Work out the finished part from the listing and answer in its coordinate system (mm). Face numbers are marked on the shaded views. A direction names the side the tool comes from. Round coordinates to 2 decimals unless told otherwise and drop trailing zeros. Write each loop counter-clockwise with the first axis right and the second up, starting at its lowest first coordinate (ties: lowest second). Pieces come first, ordered by that corner, then holes. Notation, with made-up numbers: M 49,-1.5 L 80,-1.5 A18 cw 80,9.5 Z; hole C -12,11.5 d10. An arc over 180 degrees is marked long. One line per item, written item: value. Start each with the question number.
Q1. A tool of negligible diameter and unlimited length cuts with its end or side. For the marked faces 1 and 2, from which of +Z, -Z, +X, -X, +Y, -Y can it reach the whole face along a straight path? Write none if from no direction.
Q2. Find section A-A (y = 0). Write down the section's boundary in (x, z) (3 decimals), and give its area (3 significant figures).
Q3. Consider probe 1 along Y at (x, z) = (16.51, 1.2); probe 2 along Z at (x, y) = (13, -4.75); probe 3 along X at (y, z) = (-1.25, 1.25). Determine where each line is inside the solid, lowest interval first.
Q4. Given pin 1 Ø7.5 at (y, z) = (0, 9.525) entering from +X; pin 2 Ø2 at (x, y) = (19.5, -1) entering from +Z; pin 3 Ø3 at (y, z) = (-3, 10.5) entering from +X, each flat-ended and moving along its own axis, determine where each tip first touches the part or whether it passes through.
Q5. Find section D-D (z = 2.5). Write down the section's boundary in (x, y), and give its area (3 significant figures).
Q6. Find section C-C (y = -5). Write down the section's boundary in (x, z) (3 decimals).
Q7. Find section B-B (x = 16.51). Write down the section's boundary in (y, z).
Q8. The mould has two halves that part along X. Classify the marked faces 3, 4, 5 and 6: released by +X, released by -X, zero draft, split by the parting line, or undercut.
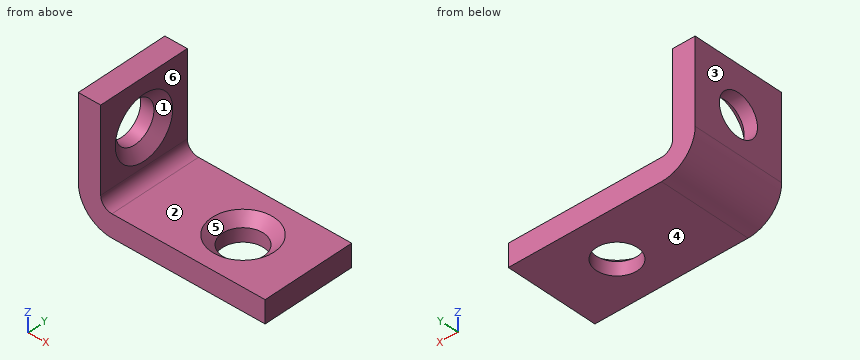
from build123d import *

# Parameters (mm, degrees)
EXTRUDE_THIN1_START = -6.35
EXTRUDE_THIN1_DEPTH = 12.7
SKETCH4_R           = 2.794
EXTRUDE3_DEPTH      = 29.141606724
SKETCH6_R           = 2.794
CUT_EXTRUDE1_DEPTH  = 31.618591166


# Read off the part's stored shape, not the designer's step: Extrude-Thin1
with BuildPart() as part:
    # Extrude-Thin1 outline → Extrude-Thin1 (new body)
    with BuildSketch(Plane(origin=(0, 0, 0), x_dir=(1, 0, 0), z_dir=(0, 1, 0)).offset(EXTRUDE_THIN1_START)):
        with BuildLine():
            Line((4.572, -3.048), (25.4, -3.048))
            Line((25.4, -3.048), (25.4, 0))
            Line((25.4, 0), (4.572, 0))
            ThreePointArc((4.572, 0), (1.339107796, -1.339107796), (0, -4.572))
            Line((0, -4.572), (0, -15.875))
            Line((0, -15.875), (3.048, -15.875))
            Line((3.048, -15.875), (3.048, -4.572))
            ThreePointArc((3.048, -4.572), (3.494369265, -3.494369265), (4.572, -3.048))
        make_face()
    extrude(amount=EXTRUDE_THIN1_DEPTH)

    # Sketch4 → Extrude3 (cut, through all)
    with BuildSketch(Plane(origin=(3.048, 0, 0), x_dir=(0, 0, -1), z_dir=(1, 0, 0))):
        with Locations((-9.525, 0)):
            Circle(SKETCH4_R)
    extrude(amount=-EXTRUDE3_DEPTH, mode=Mode.SUBTRACT)

    # Sketch6 → Cut-Extrude1 (cut, through all)
    with BuildSketch(Plane.XY):
        with Locations(Location((16.51, 0, 0), (0, 0, 180))):
            Circle(SKETCH6_R)
    extrude(amount=CUT_EXTRUDE1_DEPTH, mode=Mode.SUBTRACT)

    # Cut-Extrude2 cone 1 section (through the dimple's axis) → Cut-Extrude2 (revolve, cut)
    with BuildSketch(Plane(origin=(3.048, 0, 9.525), x_dir=(0, 0, -1), z_dir=(0, 1, 0))):
        Polygon((0, 0), (4.2164, 0), (0, 3.665260601), align=None)
    revolve(axis=Axis((3.048, 0, 9.525), (-1, 0, 0)), mode=Mode.SUBTRACT)

    # Cut-Extrude3 cone 1 section (through the dimple's axis) → Cut-Extrude3 (revolve, cut)
    with BuildSketch(Plane(origin=(16.51, 0, 3.048), x_dir=(0, -1, 0), z_dir=(1, 0, 0))):
        Polygon((0, 0), (4.2164, 0), (0, 3.665260601), align=None)
    revolve(axis=Axis((16.51, 0, 3.048), (0, 0, -1)), mode=Mode.SUBTRACT)


solid = part.part
The answers:
1. face 1: +X
1. face 2: +Z, +X, +Y, -Y
2. outline: M 0,4.572 A4.572 ccw 4.572,0 L 13.716,0 L 13.716,1.812 L 12.294,3.048 L 4.572,3.048 A1.524 cw 3.048,4.572 L 3.048,5.309 L 1.812,6.731 L 0,6.731 Z; M 0,12.319 L 1.812,12.319 L 3.048,13.741 L 3.048,15.875 L 0,15.875 Z; M 19.304,0 L 25.4,0 L 25.4,3.048 L 20.726,3.048 L 19.304,1.812 Z
2. area: 74.9 mm2
3. probe 1: -6.35 to -2.79, 2.79 to 6.35
3. probe 2: 0 to 3.05
3. probe 3: 1.43 to 14.01, 19.01 to 25.4
4. pin 1: x = 2.64
4. pin 2: z = 2.99
4. pin 3: x = 3.05
5. outline: M 0.5,-6.35 L 25.4,-6.35 L 25.4,6.35 L 0.5,6.35 Z; hole C 16.51,0 d7.17
5. area: 276 mm2
6. outline: M 0,4.572 A4.572 ccw 4.572,0 L 25.4,0 L 25.4,3.048 L 4.572,3.048 A1.524 cw 3.048,4.572 L 3.048,15.875 L 0,15.875 Z
7. outline: M -6.35,0 L -2.79,0 L -2.79,1.81 L -4.22,3.05 L -6.35,3.05 Z; M 2.79,0 L 6.35,0 L 6.35,3.05 L 4.22,3.05 L 2.79,1.81 Z
8. face 3: released by -X
8. face 4: zero draft
8. face 5: undercut
8. face 6: released by +X
